Autodesk Inventor part; units mm, degrees
ref_plane "YZ Plane" through (0, 0, 0) normal (1, 0, 0) x (0, 1, 0)
ref_plane "XZ Plane" through (0, 0, 0) normal (0, 1, 0) x (-1, 0, 0)
ref_plane "XY Plane" through (0, 0, 0) normal (0, 0, 1) x (1, 0, 0)
sketch "Szkic1" plane through (0, 0, 0) normal (0, 0, 1) x (1, 0, 0)
  line L0 (0, 0) -> (10, 0)
  line L1 (10, 0) -> (10, 10)
  line L2 (10, 10) -> (0, 10)
  line L3 (0, 10) -> (0, 0)
  dimension "d0" = 10
  dimension "d1" = 10
extrude "Wyciągnięcie proste1" add sketch "Szkic1" along normal blind 10
fillet "Zaokrąglenie1" radius 5 12 edges at (10, 10, 5) (5, 10, 10) (10, 5, 10) (10, 5, 0) (5, 0, 0) (10, 0, 5) (0, 5, 0) (5, 10, 0) (0, 10, 5) (0, 0, 5) (0, 5, 10) (5, 0, 10)
sketch "Szkic2" plane through (0, 0, 0) normal (0, 0, 1) x (1, 0, 0)
  line L0 (5, 5) -> (5, 5)
  circle A0 centre (5, 5) radius 2.6
  line L1 (5, 0) -> (5, 5)
  circle A1 centre (5, 5) radius 3.5
  point P0 (0, 0)
  dimension "d5" = 5.2
  dimension "d6" = 7
extrude "Wyciągnięcie proste2" add sketch "Szkic2" along normal blind 3.25 and the other way blind 40
properties part number "pointer"
Input: part model. Units: mm. Frame: model coordinates. Give positions to 0.01 mm unless a question says otherwise; leave off trailing zeros. Loops run counter-clockwise (first coordinate to the right, second up) from the corner with the lowest first, then second, coordinate; pieces in that order, holes last. Notation, with made-up numbers: M -7.75,18 L 20.25,18 A11 cw 20.25,30 Z; hole C 20.25,-14 d4. An arc over 180 degrees is marked long. Answer as CSV lines item,"result". Start each with the question number.
1. Pin query (flat end, axial travel): P1, Ø3, axis at y = 3.5, z = -24.5, coming from the -X side; P2, Ø4, axis at y = 8.5, z = -2.5, coming from the -X side; P3, Ø4, axis at y = 2, z = -7.5, coming from the -X side. Return the tip coordinate at first contact, or that it passes through.
2. Line query: L1, parallel to X at y = 5, z = -13; L2, parallel to X at y = 3, z = -25.5. Output: solid intervals per line, ascending.
3. Section C-C on z = -5. Return loops of the section in (x, y).
4. Pull-direction query (Y, two-part tool) for faces 1 (the face through (4.662, 7.578, -19.35)), 2 (the face through (5, 8, -40)), 3 (the face through (8.233, 6.341, -19.576)); classes: released by +Y, released by -Y, zero draft, split by the parting line, or undercut.
Computed values:
1,P1,"stops at x = 1.5"
1,P2,"stops at x = 1.84"
1,P3,"stops at x = 1.65"
2,L1,"x = 1.5 to 2.4, 7.6 to 8.5"
2,L2,"x = 2.13 to 3.34, 6.66 to 7.87"
3,outline,"C 5,5 d7; hole C 5,5 d5.2"
4,face 1,"undercut"
4,face 2,"zero draft"
4,face 3,"split by the parting line"
